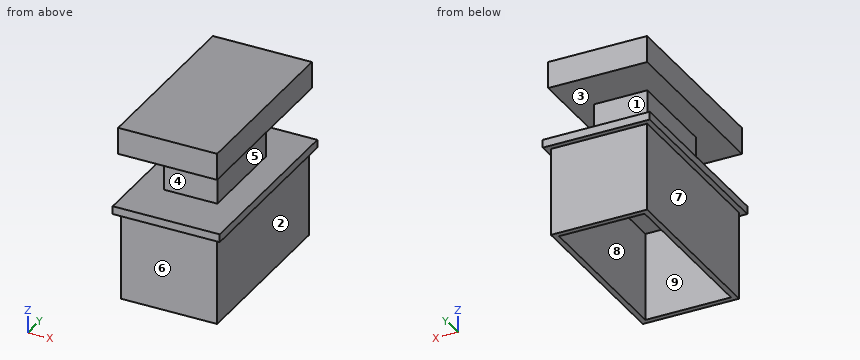
from build123d import *

# Parameters (mm, degrees)
SCHIZZO1_W                   = 4
SCHIZZO1_H                   = 7
ESTRUSIONE_ESTRUSIONE1_DEPTH = 0.3
SCHIZZO2_W                   = 3.6
SCHIZZO2_H                   = 6.6
ESTRUSIONE_ESTRUSIONE2_DEPTH = 3.3
SCHIZZO3_W                   = 3.2
SCHIZZO3_H                   = 6.2
TAGLIO_ESTRUSIONE1_DEPTH     = 4.3
SCHIZZO6_W                   = 2
SCHIZZO6_H                   = 3.5
ESTRUSIONE_ESTRUSIONE3_DEPTH = 2.3
SCHIZZO7_W                   = 3.7
SCHIZZO7_H                   = 6.8
ESTRUSIONE_ESTRUSIONE4_DEPTH = 1


with BuildPart() as part:
    # Schizzo1 → Estrusione-Estrusione1 (new body)
    with BuildSketch(Plane.XY):
        with Locations((2, 3.5)):
            Rectangle(SCHIZZO1_W, SCHIZZO1_H)
    extrude(amount=ESTRUSIONE_ESTRUSIONE1_DEPTH)

    # Schizzo2 → Estrusione-Estrusione2 (add)
    with BuildSketch(Plane.XY):
        with Locations((2, 3.5)):
            Rectangle(SCHIZZO2_W, SCHIZZO2_H)
    extrude(amount=-ESTRUSIONE_ESTRUSIONE2_DEPTH)

    # Schizzo3 → Taglio-Estrusione1 (cut, through all)
    with BuildSketch(Plane.XY):
        with Locations((2, 3.5)):
            Rectangle(SCHIZZO3_W, SCHIZZO3_H)
    extrude(amount=-TAGLIO_ESTRUSIONE1_DEPTH, mode=Mode.SUBTRACT)

    # Schizzo6 → Estrusione-Estrusione3 (add)
    with BuildSketch(Plane.XY):
        with Locations((2, 3.5)):
            Rectangle(SCHIZZO6_W, SCHIZZO6_H)
    extrude(amount=ESTRUSIONE_ESTRUSIONE3_DEPTH)

    # Schizzo7 → Estrusione-Estrusione4 (add)
    with BuildSketch(Plane.XY.offset(2.3)):
        with Locations((2, 3.5)):
            Rectangle(SCHIZZO7_W, SCHIZZO7_H)
    extrude(amount=ESTRUSIONE_ESTRUSIONE4_DEPTH)


solid = part.part
Source: CAD feature listing. Evaluate the final solid. Frame: model axes, mm. Face numbers are marked on the shaded views. A direction names the side the tool comes from. Round coordinates to 2 decimals unless told otherwise and drop trailing zeros. Loops run counter-clockwise (first coordinate to the right, second up) from the corner with the lowest first, then second, coordinate; pieces in that order, holes last. Notation, with made-up numbers: M 24.5,-9.75 L 71.5,-9.75 A34 ccw 71.5,29.25 Z; hole C 58,66 d2. An arc over 180 degrees is marked long. Return JSON: item names as keys, results as strings. Group by question number.
1. Material intervals for line 1 along Y through (x, z) = (2, -0.25); line 2 along X through (y, z) = (0.5, -0.75); line 3 along Z through (x, y) = (3.75, 5.5), sorted ascending. Write a range as from..to.
2. Section query D-D on y = 3.5. Output: boundary loops of the cut face in (x, z).
3. Section query C-C on y = 6.25. Output: boundary loops of the cut face in (x, z), and give its area (3 significant figures).
4. Pin query (flat end, axial travel): pin 1 (1.6 mm diameter, centred on x = 2, z = -2, fed in from -Y); pin 2 (1.6 mm diameter, centred on x = 1.5, z = 2, fed in from +Y); pin 3 (0.8 mm diameter, centred on x = 2.5, z = 3, fed in from -Y). Return the tip coordinate at first contact, or that it passes through.
5. Section query A-A on x = 3.5. Output: boundary loops of the cut face in (y, z), and give its area (3 significant figures).
6. Mould query, pull axis X, two halves, no side actions, for the marked faces 6, 7, 8 and 9. Classes: released by +X, released by -X, zero draft, split by the parting line, or undercut.
7. Reachability of the marked faces 1, 2, 3, 4 and 5 from +Z, -Z, +X, -X, +Y, -Y: full face, straight path, thin tool, end or side. Return the list, or none.
8. Section query B-B on z = -1.25. Output: boundary loops of the cut face in (x, y), and give its area (3 significant figures).
Checks:
{
 "1": {"line 1": "y = 0.2..0.4, 6.6..6.8", "line 2": "x = 0.2..0.4, 3.6..3.8", "line 3": "z = -3.3..0.3, 2.3..3.3"},
 "2": {"outline": "M 0,0 L 0.2,0 L 0.2,-3.3 L 0.4,-3.3 L 0.4,0 L 3.6,0 L 3.6,-3.3 L 3.8,-3.3 L 3.8,0 L 4,0 L 4,0.3 L 3,0.3 L 3,2.3 L 3.85,2.3 L 3.85,3.3 L 0.15,3.3 L 0.15,2.3 L 1,2.3 L 1,0.3 L 0,0.3 Z"},
 "3": {"outline": "M 0,0 L 0.2,0 L 0.2,-3.3 L 0.4,-3.3 L 0.4,0 L 3.6,0 L 3.6,-3.3 L 3.8,-3.3 L 3.8,0 L 4,0 L 4,0.3 L 0,0.3 Z; M 0.15,2.3 L 3.85,2.3 L 3.85,3.3 L 0.15,3.3 Z", "area": "6.22 mm²"},
 "4": {"pin 1": "stops at y = 0.2", "pin 2": "stops at y = 6.9", "pin 3": "stops at y = 0.1"},
 "5": {"outline": "M 0,0 L 0.2,0 L 0.2,-3.3 L 0.4,-3.3 L 0.4,0 L 6.6,0 L 6.6,-3.3 L 6.8,-3.3 L 6.8,0 L 7,0 L 7,0.3 L 0,0.3 Z; M 0.1,2.3 L 6.9,2.3 L 6.9,3.3 L 0.1,3.3 Z", "area": "10.2 mm²"},
 "6": {"face 6": "zero draft", "face 7": "released by -X", "face 8": "undercut", "face 9": "undercut"},
 "7": {"face 1": "+X, -X, +Y", "face 2": "-Z, +X, +Y, -Y", "face 3": "none", "face 4": "+X, -X, -Y", "face 5": "+X, +Y, -Y"},
 "8": {"outline": "M 0.2,0.2 L 3.8,0.2 L 3.8,6.8 L 0.2,6.8 Z; hole M 0.4,0.4 L 3.6,0.4 L 3.6,6.6 L 0.4,6.6 Z", "area": "3.92 mm²"}
}
